```python
from build123d import *

# Parameters (mm, degrees)
SKETCH1_W             = 325
SKETCH1_H             = 103
BOSS_EXTRUDE1_DEPTH   = 165
M6_TAPPED_HOLE1_D     = 5
M6_TAPPED_HOLE1_DEPTH = 15
M6_TAPPED_HOLE1_TIP   = 1.502151548
CUT_EXTRUDE1_DEPTH    = 35


with BuildPart() as part:
    # Sketch1 → Boss-Extrude1 (new body)
    with BuildSketch(Plane(origin=(0, 0, 0), x_dir=(1, 0, 0), z_dir=(0, 1, 0))):
        with Locations((162.5, 51.5)):
            Rectangle(SKETCH1_W, SKETCH1_H)
    extrude(amount=BOSS_EXTRUDE1_DEPTH)

    # M6 Tapped Hole1
    with Locations(Plane(origin=(0, 165, 0), x_dir=(1, 0, 0), z_dir=(0, 1, 0))):
        with Locations((310, 51.5), (258, 51.5), (206, 51.5), (154, 51.5)):
            Hole(M6_TAPPED_HOLE1_D / 2, depth=M6_TAPPED_HOLE1_DEPTH)
            with Locations((0, 0, -(M6_TAPPED_HOLE1_DEPTH + M6_TAPPED_HOLE1_TIP / 2))):  # 118° drill point
                Cone(0, M6_TAPPED_HOLE1_D / 2, M6_TAPPED_HOLE1_TIP, mode=Mode.SUBTRACT)

    # Sketch5 → Cut-Extrude1 (cut)
    with BuildSketch(Plane.XZ):
        with BuildLine():
            Line((50, 0), (50, -11.5))
            ThreePointArc((50, -11.5), (53.5, -15), (57, -11.5))
            Line((57, -11.5), (57, 0))
            Line((57, 0), (50, 0))
        make_face()
        with BuildLine():
            Line((247, 0), (247, -11.5))
            ThreePointArc((247, -11.5), (243.5, -15), (240, -11.5))
            Line((240, -11.5), (240, 0))
            Line((240, 0), (247, 0))
        make_face()
        with BuildLine():
            Line((247, -103), (240, -103))
            Line((240, -103), (240, -91.5))
            ThreePointArc((240, -91.5), (243.5, -88), (247, -91.5))
            Line((247, -91.5), (247, -103))
        make_face()
        with BuildLine():
            Line((50, -103), (50, -91.5))
            ThreePointArc((50, -91.5), (53.5, -88), (57, -91.5))
            Line((57, -91.5), (57, -103))
            Line((57, -103), (50, -103))
        make_face()
    extrude(amount=-CUT_EXTRUDE1_DEPTH, mode=Mode.SUBTRACT)


solid = part.part
```
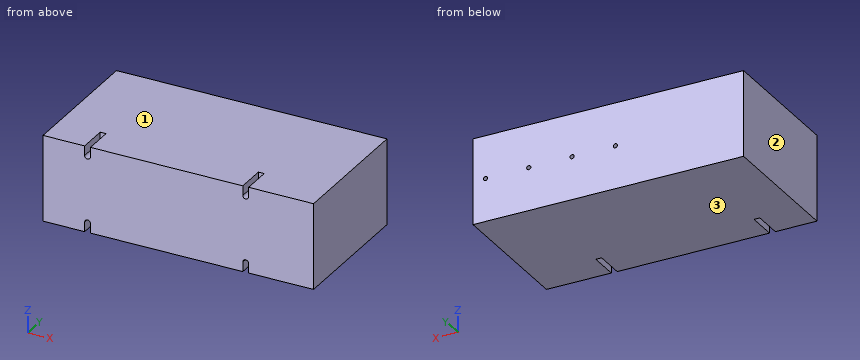
Here's how the part is built. I have some questions about the finished solid (model axes, mm). Face numbers are marked on the shaded views. Give positions to 0.01 mm unless a question says otherwise; leave off trailing zeros. Put each result on its own line as item: value. Start each with the question number.
(1) Will these pins go through, and if not, where does the flat tip stop? pin 1 Ø12.5 at (y, z) = (19, -95) entering from -X; pin 2 Ø2 at (x, z) = (244, -92.5) entering from -Y; pin 3 Ø4.5 at (x, z) = (258, -51.5) entering from +Y.
(2) If we mould it in two halves opening along Z, with no side actions, what happens to the marked faces 1, 2 and 3? For each: +Z half, -Z half, draft (parallel to the pull), parting line (faces both ways), or undercut.
(3) I need wall thicknesses on line 1 along X through (y, z) = (161, -51.5); line 2 along X through (y, z) = (159, -51); line 3 along Z through (x, y) = (258, 156). Which ranges of each line are inside material? Lowest first, please. Write a range as [from, to].
Answer block:
1. pin 1: x = 0
1. pin 2: y = 35
1. pin 3: y = 149.85
2. face 1: +Z half
2. face 2: draft
2. face 3: -Z half
3. line 1: [0, 151.5], [156.5, 203.5], [208.5, 255.5], [260.5, 307.5], [312.5, 325]
3. line 2: [0, 151.55], [156.45, 203.55], [208.45, 255.55], [260.45, 307.55], [312.45, 325]
3. line 3: [-103, -54], [-49, 0]
